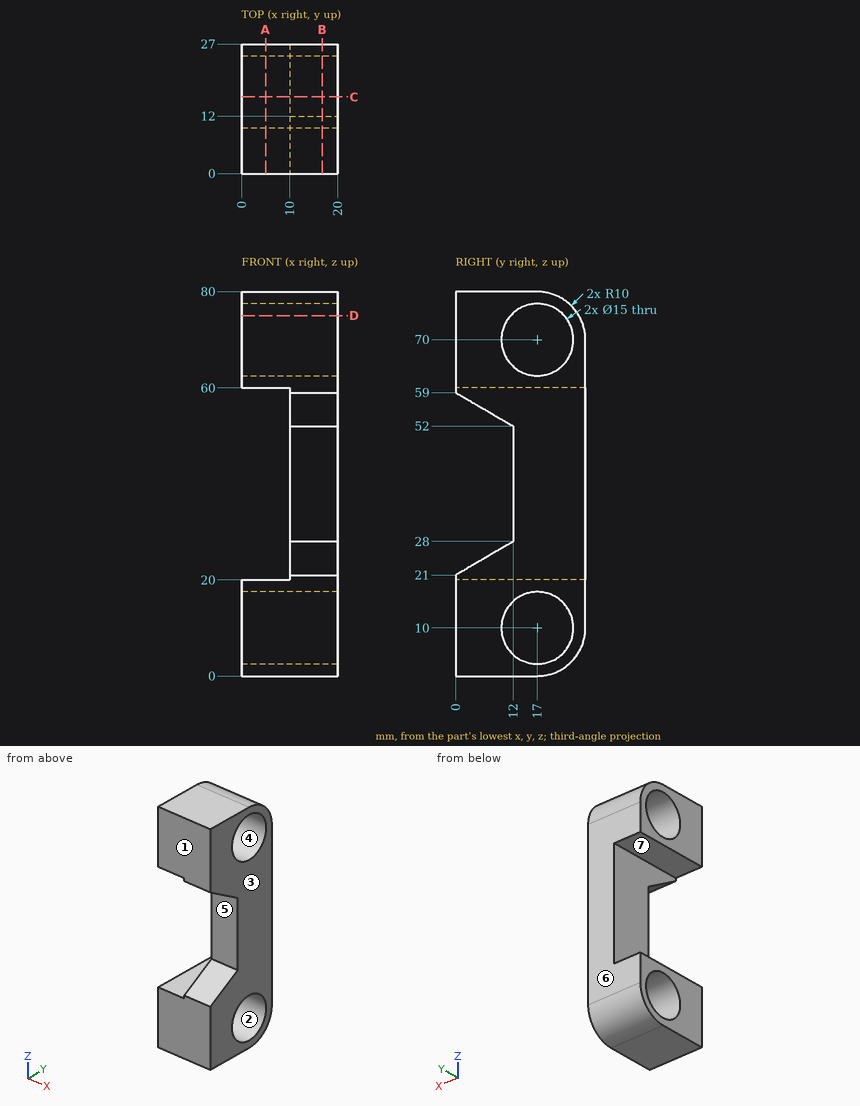
Can you work these out from the drawing? Everything is in mm from the part's minimum corner. A direction names the side the tool comes from. Give positions to 0.01 mm unless a question says otherwise; leave off trailing zeros. Order: outer loops, then holes, each group sorted by start corner. A loop starts at its lowest first (then second) coordinate and runs counter-clockwise, first axis right, second up.
1. Suppose I cut it at C-C (y = 16). List the corners of the cut face in (x, z) for me, plus the area to 3 significant figures.
2. Suppose I cut it at D-D (z = 75). List the corners of the cut face in (x, y) for me, plus the area to 3 significant figures.
3. For the marked faces 5, 6 and 7, which set-ups out of +Z, -Z, +X, -X, +Y, -Y let a thin tool reach every point of the face, with its end or its side?
4. Suppose I cut it at B-B (x = 16.75). List the corners of the cut face in (y, z) for me.
5. Suppose I cut it at A-A (x = 5). List the corners of the cut face in (y, z) for me, plus the area to 3 significant figures.
6. I need wall thicknesses on L1, parallel to Y at x = 14.5, z = 10; L2, parallel to Z at x = 5, y = 18; L3, parallel to X at y = 10, z = 26. Which ranges of each line are inside material? Lowest first, please.
7. We'd pull the mould along Y, two halves only. Please class the marked faces 1, 2, 3 and 4: pulls with the +Y half, pulls with the -Y half, needs draft (parallel to the pull), parting line crosses it, or undercut.
8. Will these pins go through, and if not, where does the flat tip stop? P1, Ø13.5, axis at y = 17, z = 70, coming from the +X side; P2, Ø1, axis at x = 17, z = 45, coming from the -Y side; P3, Ø13.5, axis at y = 13.5, z = 30.5, coming from the -X side.
Solved:
1. outline: (0, 0) - (20, 0) - (20, 2.57) - (0, 2.57) - close; (0, 17.43) - (20, 17.43) - (20, 62.57) - (0, 62.57) - (0, 60) - (10, 60) - (10, 20) - (0, 20) - close; (0, 77.43) - (20, 77.43) - (20, 80) - (0, 80) - close
1. area: 605 mm2
2. outline: (0, 0) - (20, 0) - (20, 11.41) - (0, 11.41) - close; (0, 22.59) - (20, 22.59) - (20, 25.66) - (0, 25.66) - close
2. area: 290 mm2
3. face 5: +X, -X, -Y
3. face 6: +Z, -Z, +X, -X, +Y
3. face 7: -X, +Y, -Y
4. outline: (0, 0) - (17, 0) arc R10 ccw to (27, 10) - (27, 70) arc R10 ccw to (17, 80) - (0, 80) - (0, 59) - (12, 52) - (12, 28) - (0, 21) - close; hole circle Ø15 at (17, 10); hole circle Ø15 at (17, 70)
5. outline: (0, 0) - (17, 0) arc R10 ccw to (27, 10) - (27, 20) - (0, 20) - close; (0, 60) - (27, 60) - (27, 70) arc R10 ccw to (17, 80) - (0, 80) - close; hole circle Ø15 at (17, 10); hole circle Ø15 at (17, 70)
5. area: 684 mm2
6. L1: y = 0 to 9.5, 24.5 to 27
6. L2: z = 0.05 to 2.57, 17.43 to 20, 60 to 62.57, 77.43 to 79.95
6. L3: x = 10 to 20
7. face 1: pulls with the -Y half
7. face 2: undercut
7. face 3: needs draft
7. face 4: undercut
8. P1: passes through
8. P2: stops at y = 12
8. P3: stops at x = 10
